Check sheet for the modelled part. Datum: model origin and axes. Units: mm. A direction names the side the tool comes from. Coordinates: 2 decimals unless noted, no trailing zeros. Order: outer loops, then holes, each group sorted by start corner. A loop starts at its lowest first (then second) coordinate and runs counter-clockwise, first axis right, second up.
1. Cross-section at C-C (x = 3). Enter the section's corners in (y, z).
2. Thickness scan on line 1 (X direction, y = -4.1, z = 0); line 2 (Y direction, x = 1, z = -10); line 3 (Z direction, x = -1.5, y = -4.05). Record the ranges inside material, lowest first.
3. Set-up check for faces 1 (the cylindrical face through (-2.44, -4.21, 0.54)), 2 (the flat face through (1, -1, 1)), 3 (the cylindrical face through (0, -1, -16)): record each of +Z, -Z, +X, -X, +Y, -Y from which the full face is reachable in a straight line by a thin tool's end or side.
4. Cross-section at A-A (z = 0). Enter the section's corners in (x, y).
5. Cross-section at D-D (z = -4.75). Enter the section's corners in (x, y), then the cut area to 3 significant figures.
6. Gauge pin test, flat end, axial feed: pin 1 Ø4 at (x, z) = (0, 0) entering from -Y. Record the tip position at first contact, or that the pin passes through.
7. Cross-section at B-B (y = -1.6). Enter the section's corners in (x, z), then the cut area to 3 significant figures.
8. Draft check along X on faces 4 (the flat face through (-2.32, -0.69, -8.23)), 5 (the cylindrical face through (0.691, -0.493, 2.194)), 6 (the flat face through (0, -5.2, -3)), 7 (the cylindrical face through (0.33, -2.08, 1.05)). Enter one of: released by +X, released by -X, zero draft, split by the parting line, or undercut.
```python
from build123d import *

# Parameters (mm, degrees)
BOSS_EXTRUDE1_DEPTH = 1.4
SKETCH2_R           = 3.5
BOSS_EXTRUDE2_DEPTH = 3.8
SKETCH3_R           = 2.3
CUT_EXTRUDE1_DEPTH  = 1
SKETCH4_R           = 2.5
CUT_EXTRUDE2_DEPTH  = 2
CUT_EXTRUDE3_REACH  = 18.908
SKETCH5_R           = 1.102182


with BuildPart() as part:
    # Sketch1 → Boss-Extrude1 (new body)
    with BuildSketch(Plane(origin=(0, 0, 0), x_dir=(1, 0, 0), z_dir=(0, 1, 0))):
        with BuildLine():
            ThreePointArc((2, 14), (0, 16), (-2, 14))
            Line((-2, 14), (-2.65, 2.286373))
            ThreePointArc((-2.65, 2.286373), (-2.286373, -2.65), (2.65, -2.286373))
            ThreePointArc((2.65, -2.286373), (3.5, 0), (2.65, 2.286373))
            Line((2.65, 2.286373), (2, 14))
        make_face()
        with BuildLine():
            ThreePointArc((0, 3.8), (-0.6, 4.4), (0, 5))
            ThreePointArc((0, 5), (0.424264, 4.824264), (0.6, 4.4))
            ThreePointArc((0.6, 4.4), (0.424264, 3.975736), (0, 3.8))
        make_face(mode=Mode.SUBTRACT)
        with BuildLine():
            ThreePointArc((0, 5.8), (-0.6, 6.4), (0, 7))
            ThreePointArc((0, 7), (0.424264, 6.824264), (0.6, 6.4))
            ThreePointArc((0.6, 6.4), (0.424264, 5.975736), (0, 5.8))
        make_face(mode=Mode.SUBTRACT)
        with BuildLine():
            ThreePointArc((0, 7.8), (-0.6, 8.4), (0, 9))
            ThreePointArc((0, 9), (0.424264, 8.824264), (0.6, 8.4))
            ThreePointArc((0.6, 8.4), (0.424264, 7.975736), (0, 7.8))
        make_face(mode=Mode.SUBTRACT)
        with BuildLine():
            ThreePointArc((0, 9.8), (-0.6, 10.4), (0, 11))
            ThreePointArc((0, 11), (0.424264, 10.824264), (0.6, 10.4))
            ThreePointArc((0.6, 10.4), (0.424264, 9.975736), (0, 9.8))
        make_face(mode=Mode.SUBTRACT)
        with BuildLine():
            ThreePointArc((0, 11.8), (-0.6, 12.4), (0, 13))
            ThreePointArc((0, 13), (0.424264, 12.824264), (0.6, 12.4))
            ThreePointArc((0.6, 12.4), (0.424264, 11.975736), (0, 11.8))
        make_face(mode=Mode.SUBTRACT)
        with BuildLine():
            ThreePointArc((0.6, 14.4), (0.424264, 13.975736), (0, 13.8))
            ThreePointArc((0, 13.8), (-0.424264, 14.824264), (0.6, 14.4))
        make_face(mode=Mode.SUBTRACT)
    extrude(amount=-BOSS_EXTRUDE1_DEPTH)

    # Sketch2 → Boss-Extrude2 (add)
    with BuildSketch(Plane(origin=(0, -1.4, 0), x_dir=(-1, 0, 0), z_dir=(0, -1, 0))):
        with Locations(Location((0, 0, 0), (0, 0, 139.212962))):
            Circle(SKETCH2_R)
    extrude(amount=BOSS_EXTRUDE2_DEPTH)

    # Sketch3 → Cut-Extrude1 (cut)
    with BuildSketch(Plane(origin=(0, 0, 0), x_dir=(1, 0, 0), z_dir=(0, 1, 0))):
        with Locations(Location((0, 0, 0), (0, 0, 270))):
            Circle(SKETCH3_R)
    extrude(amount=-CUT_EXTRUDE1_DEPTH, mode=Mode.SUBTRACT)

    # Sketch4 → Cut-Extrude2 (cut)
    with BuildSketch(Plane(origin=(0, -5.2, 0), x_dir=(-1, 0, 0), z_dir=(0, -1, 0))):
        with Locations(Location((0, 0, 0), (0, 0, 90))):
            Circle(SKETCH4_R)
    extrude(amount=-CUT_EXTRUDE2_DEPTH, mode=Mode.SUBTRACT)

    # Sketch5 → Cut-Extrude3 (cut, up to next)
    with BuildSketch(Plane(origin=(0, -1, 0), x_dir=(1, 0, 0), z_dir=(0, 1, 0)), mode=Mode.PRIVATE) as cut_extrude3_sk1:
        with Locations(Location((0, 0, 0), (0, 0, 270))):
            Circle(SKETCH5_R)
    cut_extrude3_tool1 = extrude(cut_extrude3_sk1.sketch, amount=-CUT_EXTRUDE3_REACH, mode=Mode.PRIVATE) & part.part
    add(cut_extrude3_tool1.solids().sort_by_distance((0, -1, 0))[0], mode=Mode.SUBTRACT)


solid = part.part
```
Data:
1. outline: (-5.2, -1.8) - (0, -1.8) - (0, 1.8) - (-5.2, 1.8) - close
2. line 1: x = -3.5 to -2.5, 2.5 to 3.5
2. line 2: y = -1.4 to 0
2. line 3: z = -3.16 to -2, 2 to 3.16
3. face 1: -Y
3. face 2: +Y
3. face 3: -Z, +Y, -Y
4. outline: (-3.5, -5.2) - (-2.5, -5.2) - (-2.5, -3.2) - (-1.1, -3.2) - (-1.1, -1) - (-2.3, -1) - (-2.3, 0) - (-3.5, 0) - close; (1.1, -3.2) - (2.5, -3.2) - (2.5, -5.2) - (3.5, -5.2) - (3.5, 0) - (2.3, 0) - (2.3, -1) - (1.1, -1) - close
5. outline: (-2.51, -1.4) - (-0.49, -1.4) - (-0.49, 0) - (-2.51, 0) - close; (0.49, -1.4) - (2.51, -1.4) - (2.51, 0) - (0.49, 0) - close
5. area: 5.67 mm2
6. pin 1: stops at y = -3.2
7. outline: circle Ø7 at (0, 0); hole circle Ø2.2 at (0, 0)
7. area: 34.7 mm2
8. face 4: released by -X
8. face 5: undercut
8. face 6: zero draft
8. face 7: undercut
